The model under review builds one solid part; all positions refer to its coordinate system, in mm. A direction names the side the tool comes from. Round coordinates to 2 decimals unless told otherwise and drop trailing zeros. Order: outer loops, then holes, each group sorted by start corner. A loop starts at its lowest first (then second) coordinate and runs counter-clockwise, first axis right, second up. Notation, with made-up numbers: M 56.5,26.5 L 104.5,26.5 A26 ccw 104.5,52.5 Z; hole C -31,64.25 d5. An arc over 180 degrees is marked long. One line per item, written item: value. Start each with the question number.
from build123d import *

# Parameters (mm, degrees)
SKETCH_W       = 70
SKETCH_H       = 70
PAD_DEPTH      = 10
SKETCH001_R    = 32
SKETCH001_R_2  = 27
POCKET_DEPTH   = 5
SKETCH003_R    = 2.25
HOLE_DEPTH     = 10
HOLE_TIPS_R    = 2.25
SKETCH004_R    = 2.25
HOLE001_DEPTH  = 10
HOLE001_TIPS_R = 2.25


with BuildPart() as part:
    # Sketch → Pad (new body)
    with BuildSketch(Plane.XZ):
        Rectangle(SKETCH_W, SKETCH_H)
    extrude(amount=PAD_DEPTH)

    # Sketch001 (on Face6 of Pad) → Pocket (cut)
    with BuildSketch(Plane.XZ.offset(10)):
        Circle(SKETCH001_R)
        Circle(SKETCH001_R_2, mode=Mode.SUBTRACT)
    extrude(amount=-POCKET_DEPTH, mode=Mode.SUBTRACT)

    # Sketch003 (on Face3 of Pocket) → Hole (cut)
    with BuildSketch(Plane(origin=(35, 0, 0), x_dir=(0, 0, 1), z_dir=(1, 0, 0))):
        with Locations((25, 5)):
            Circle(SKETCH003_R)
    extrude(amount=-HOLE_DEPTH, mode=Mode.SUBTRACT)

    # Hole tips → Hole tip 1 section 0
    with BuildSketch(Plane(origin=(25, 0, 0), x_dir=(0, 0, 1), z_dir=(1, 0, 0)), mode=Mode.PRIVATE) as hole_tip_1_s0:
        with Locations((25, 5)):
            Circle(HOLE_TIPS_R)
    loft([hole_tip_1_s0.sketch, Vertex(23.648064, -5, 25)], mode=Mode.SUBTRACT)

    # Sketch004 (on Face6 of Hole) → Hole001 (cut)
    with BuildSketch(Plane(origin=(0, 0, -35), x_dir=(1, 0, 0), z_dir=(0, 0, -1))):
        with Locations((-25, 5)):
            Circle(SKETCH004_R)
    extrude(amount=-HOLE001_DEPTH, mode=Mode.SUBTRACT)

    # Hole001 tips → Hole001 tip 1 section 0
    with BuildSketch(Plane(origin=(0, 0, -25), x_dir=(1, 0, 0), z_dir=(0, 0, -1)), mode=Mode.PRIVATE) as hole001_tip_1_s0:
        with Locations((-25, 5)):
            Circle(HOLE001_TIPS_R)
    loft([hole001_tip_1_s0.sketch, Vertex(-25, -5, -23.648064)], mode=Mode.SUBTRACT)


solid = part.part
Item 1: Wall thickness on L1, parallel to Z at x = 0, y = -8.6; L2, parallel to Y at x = -25, z = -31; L3, parallel to Z at x = -6, y = -6.5: over which ranges is each line inside the solid? List them lowest first.
Item 2: The part is to be moulded in two halves that separate along Y. For faces 3 (the cylindrical face through (-22.854, -5.676, -30.07)), 4 (the cylindrical face through (30.07, -5.676, 27.146)), 5 (the flat face through (-35, -5, 0)), 6 (the flat face through (-16, -10, -28)), say which applies: pulls with the +Y half, pulls with the -Y half, needs draft (parallel to the pull), parting line crosses it, or undercut.
Item 3: Machinability: for faces 1 (the cylindrical face through (-5.85, -7.54, -26.36)), 2 (the flat face through (0, 0, 0)), which of the approach directions +Z, -Z, +X, -X, +Y, -Y give a long, thin tool a straight path to every point of the face, cutting with its end or side? Answer none if there is none.
Item 4: Consider section C-C, the plane x = 0. Give the boundary of the cut face in (y, z), then the cut area to 3 significant figures.
Item 5: Consider section B-B, the plane z = 0. Give the boundary of the cut face in (x, y), then the cut area to 3 significant figures.
Item 6: Clearance check with flat-ended pins moving along their axes: P1, Ø3.5, axis at y = -5, z = 25, coming from the +X side; P2, Ø12, axis at x = 13, z = -8.5, coming from the +Y side. State where each tip first meets the part, or that it passes through.
Item 7: Consider section A-A, the plane y = -9. Give the boundary of the cut face in (x, z).
Computed:
1. L1: z = -35 to -32, -27 to 27, 32 to 35
1. L2: y = -10 to -7.25, -2.75 to 0
1. L3: z = -35 to -31.43, -26.32 to 26.32, 31.43 to 35
2. face 3: undercut
2. face 4: undercut
2. face 5: needs draft
2. face 6: pulls with the -Y half
3. face 1: -Y
3. face 2: +Z, -Z, +X, -X, +Y
4. outline: M -10,-35 L 0,-35 L 0,35 L -10,35 L -10,32 L -5,32 L -5,27 L -10,27 L -10,-27 L -5,-27 L -5,-32 L -10,-32 Z
4. area: 650 mm^2
5. outline: M -35,-10 L -32,-10 L -32,-5 L -27,-5 L -27,-10 L 27,-10 L 27,-5 L 32,-5 L 32,-10 L 35,-10 L 35,0 L -35,0 Z
5. area: 650 mm^2
6. P1: stops at x = 24.7
6. P2: stops at y = 0
7. outline: M -35,-35 L 35,-35 L 35,35 L -35,35 Z; C 0,0 d54; hole C 0,0 d64
